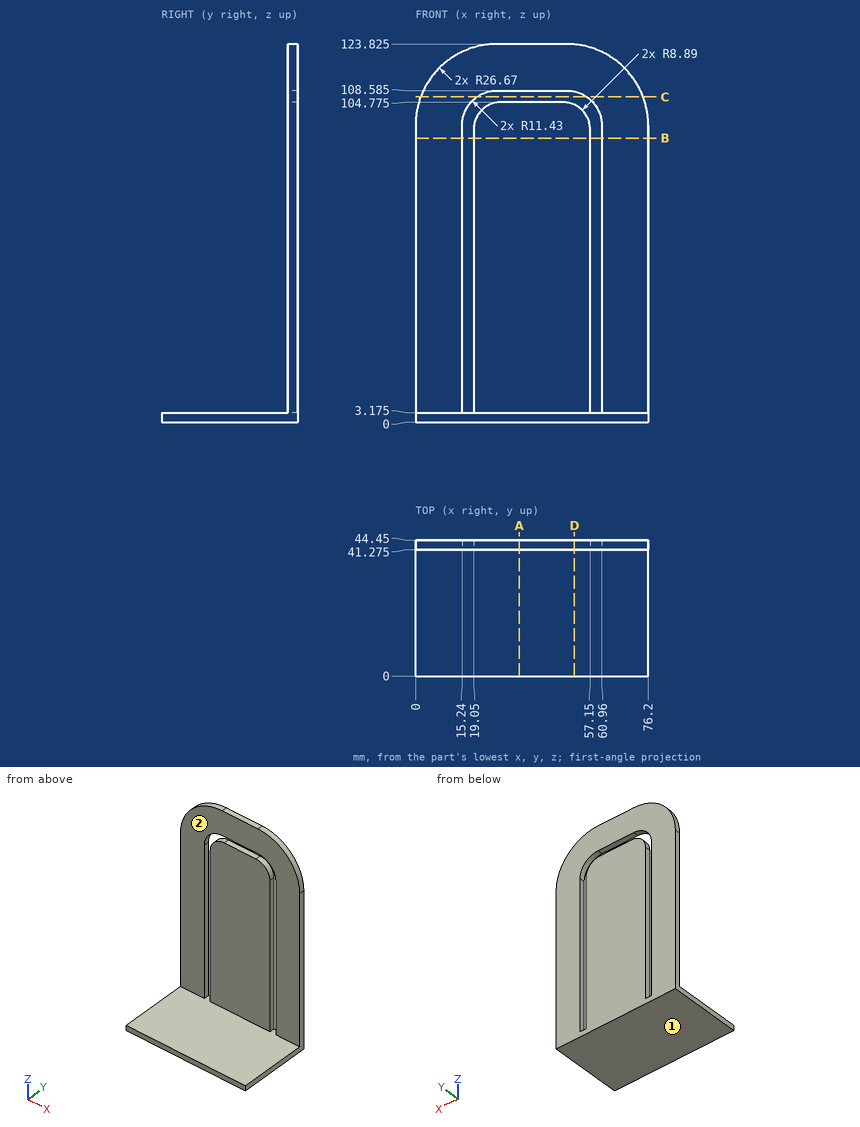
Design review of the part shown in the three views and the two pictorial views. Dimensions are in mm from the part's minimum x, y and z. A direction names the side the tool comes from. Round coordinates to 2 decimals unless told otherwise and drop trailing zeros. Order: outer loops, then holes, each group sorted by start corner. A loop starts at its lowest first (then second) coordinate and runs counter-clockwise, first axis right, second up.
Item 1: Add section C-C, the plane z = 106.5. State the section outline as (x, y) points (3 decimals), and give its area (3 significant figures).
Working result:
outline: (1.691, 41.275) - (20.089, 41.275) - (20.089, 44.45) - (1.691, 44.45) - close; (56.111, 41.275) - (74.509, 41.275) - (74.509, 44.45) - (56.111, 44.45) - close
area: 117 mm2
Item 2: Add section D-D, the plane x = 52. State the section outline as (y, z) points (3 decimals), and give its area (3 significant figures).
Working result:
outline: (0, 0) - (44.45, 0) - (44.45, 103.95) - (41.275, 103.95) - (41.275, 3.175) - (0, 3.175) - close; (41.275, 108.315) - (44.45, 108.315) - (44.45, 123.71) - (41.275, 123.71) - close
area: 510 mm2
Item 3: To check wall thickness, follow probe 1 along X at (y, z) = (41.5, 79); probe 2 along Y at (x, z) = (65.5, 47) (3 decimals); probe 3 along Z at (x, y) = (43.5, 9.5) (3 decimals). State the ranges of each line that lie inside material, in increasing order.
Working result:
probe 1: x = 0 to 15.24, 19.05 to 57.15, 60.96 to 76.2
probe 2: y = 41.275 to 44.45
probe 3: z = 0 to 3.175
Item 4: Add section A-A, the plane x = 34. State the section outline as (y, z) points (3 decimals).
Working result:
outline: (0, 0) - (44.45, 0) - (44.45, 104.775) - (41.275, 104.775) - (41.275, 3.175) - (0, 3.175) - close; (41.275, 108.585) - (44.45, 108.585) - (44.45, 123.825) - (41.275, 123.825) - close
Item 5: Machinability: for the marked faces 1 and 2, which of the approach directions +Z, -Z, +X, -X, +Y, -Y give a long, thin tool a straight path to every point of the face, cutting with its end or side? Answer none if there is none.
Working result:
face 1: -Z, +X, -X, +Y, -Y
face 2: +Z, +X, -X, -Y
Item 6: For pin 1 (23 mm diameter, centred on x = 21, z = 74.5, fed in from -Y) (3 decimals); pin 2 (3.5 mm diameter, centred on x = 33.5, y = 43, fed in from -Z); pin 3 (3 mm diameter, centred on x = 20, y = 23, fed in from +Z) (3 decimals), all flat-tipped, find the tip position at first contact; note any pin that passes through.
Working result:
pin 1: stops at y = 41.275
pin 2: stops at z = 0
pin 3: stops at z = 3.175
Item 7: Add section B-B, the plane z = 93. State the section outline as (x, y) points (3 decimals), and give its area (3 significant figures).
Working result:
outline: (0, 41.275) - (15.24, 41.275) - (15.24, 44.45) - (0, 44.45) - close; (19.05, 41.275) - (57.15, 41.275) - (57.15, 44.45) - (19.05, 44.45) - close; (60.96, 41.275) - (76.2, 41.275) - (76.2, 44.45) - (60.96, 44.45) - close
area: 218 mm2
